Could you check a few things on this model? Use its own coordinates, in mm. Face numbers are marked on the shaded views. A direction names the side the tool comes from. Give positions to 0.01 mm unless a question says otherwise; leave off trailing zeros. Loops run counter-clockwise (first coordinate to the right, second up) from the corner with the lowest first, then second, coordinate; pieces in that order, holes last. Notation, with made-up numbers: M 60.25,9.5 L 65.25,9.5 A14 cw 65.25,33.5 Z; hole C 52,26 d9. An arc over 180 degrees is marked long. Answer in a Markdown table with one row per item. Add a question column.
1. Which directions (+Z, -Z, +X, -X, +Y, -Y) give clear straight access to the entire face, cutting with the end or side of a thin tool? Please do the marked faces 4, 5 and 6.
2. Thinking about a two-plate mould opening in X: for the marked faces 1, 2 and 3, which applies, released by +X, released by -X, zero draft, split by the parting line, or undercut?
3. I'm going to push flat-ended pins straight in: pin 1 Ø6 at (x, y) = (479.5, 238.5) entering from -Z; pin 2 Ø18.5 at (x, z) = (539, 98) entering from +Y; pin 3 Ø6 at (x, z) = (356.5, 119.5) entering from -Y. Where does each tip first touch, or does it pass through?
4. If we section it at A-A on y = 0: Count the separate pieces of the cut face and the enclosed holes in it, then the cut area to 3 significant figures.
5. If we section it at C-C on z = -403.5: List the corners of the cut face in (x, y) for me.
6. I need wall thicknesses on line 1 along Y through (x, z) = (644, -10); line 2 along Y through (x, z) = (561, -145); line 3 along X through (y, z) = (97, 489). Which ranges of each line are inside material? Lowest first, please. Write a range as from..to.
7. If we section it at B-B on x = 313: List the corners of the cut face in (y, z) for me.
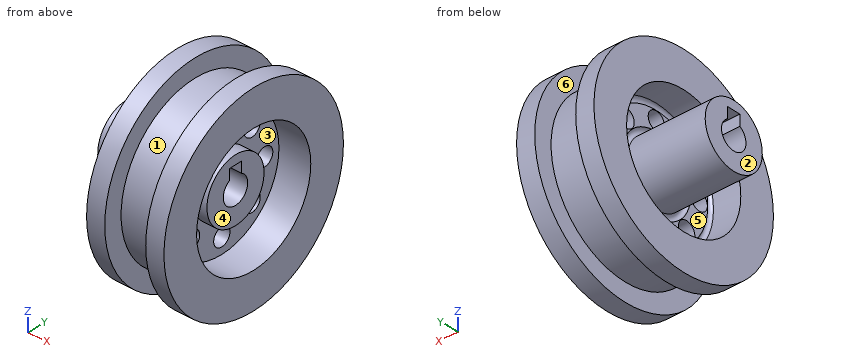
```python
from build123d import *

# Parameters (mm, degrees)
F3_DEPTH = 711.201
F5_D     = 101.6


with BuildPart() as f1:
    # F0 (on Front) → F1 (revolve)
    with BuildSketch(Plane.XZ):
        with BuildLine():
            Line((801.302386, -76.2), (191.702386, -76.2))
            Line((191.702386, -76.2), (191.702386, -177.8))
            Line((191.702386, -177.8), (623.502386, -177.8))
            ThreePointArc((623.502386, -177.8), (641.304548, -195.602162), (623.502386, -213.404324))
            Line((623.502386, -213.404324), (623.502386, -319.995676))
            ThreePointArc((623.502386, -319.995676), (641.304548, -337.797838), (623.502386, -355.6))
            Line((623.502386, -355.6), (471.102386, -355.6))
            Line((471.102386, -355.6), (471.102386, -558.8))
            Line((471.102386, -558.8), (572.702386, -558.8))
            Line((572.702386, -558.8), (572.702386, -457.2))
            Line((572.702386, -457.2), (801.302386, -457.2))
            Line((801.302386, -457.2), (801.302386, -558.8))
            Line((801.302386, -558.8), (902.902386, -558.8))
            Line((902.902386, -558.8), (902.902386, -355.6))
            Line((902.902386, -355.6), (725.102386, -355.6))
            Line((725.102386, -355.6), (725.102386, -177.8))
            Line((725.102386, -177.8), (801.302386, -177.8))
            Line((801.302386, -177.8), (801.302386, -76.2))
        make_face()
    revolve(axis=Axis((352.317811, 0, 0), (1, 0, 0)))

    # F2 (on face) → F3 (cut, through all)
    with BuildSketch(Plane(origin=(191.702386, 0, 0), x_dir=(0, -1, 0), z_dir=(-1, 0, 0))):
        with BuildLine():
            Line((38.1, 127), (0, 127))
            Line((0, 127), (-38.1, 127))
            Line((-38.1, 127), (-38.1, 65.991136))
            ThreePointArc((-38.1, 65.991136), (0, 76.2), (38.1, 65.991136))
            Line((38.1, 65.991136), (38.1, 127))
        make_face()
    extrude(amount=-F3_DEPTH, mode=Mode.SUBTRACT)

    # F5 (through all)
    with Locations(Plane(origin=(0, 0, 0), x_dir=(0, 1, 0), z_dir=(-1, 0, 0))):
        with Locations((0, 266.7), (188.585379, 188.585379), (266.7, 0), (188.585379, -188.585379), (0, -266.7), (-188.585379, -188.585379), (-266.7, 0), (-188.585379, 188.585379)):
            Hole(F5_D / 2)


solid = f1.part
```
Results:
| question | item | result |
|---|---|---|
| 1 | face 4 | +X |
| 1 | face 5 | -X |
| 1 | face 6 | none |
| 2 | face 1 | undercut |
| 2 | face 2 | released by -X |
| 2 | face 3 | released by +X |
| 3 | pin 1 | z = -506.75 |
| 3 | pin 2 | y = 551.71 |
| 3 | pin 3 | y = -134.32 |
| 4 | separate pieces | 4 |
| 4 | enclosed holes | 0 |
| 4 | area | 235,000 mm2 |
| 5 | outline | M 471.1,-386.58 L 572.7,-386.58 L 572.7,-214.99 L 801.3,-214.99 L 801.3,-386.58 L 902.9,-386.58 L 902.9,386.58 L 801.3,386.58 L 801.3,214.99 L 572.7,214.99 L 572.7,386.58 L 471.1,386.58 Z |
| 6 | line 1 | -457.09..-316.51, -216.89..-75.54, 75.54..216.89, 316.51..457.09 |
| 6 | line 2 | -539.66..-324.69, -102.9..102.9, 324.69..539.66 |
| 6 | line 3 | 471.1..572.7, 801.3..902.9 |
| 7 | outline | C 0,0 d355.6; hole M -38.1,65.99 A76.2 ccw long 38.1,65.99 L 38.1,127 L -38.1,127 Z |
